from build123d import *

# Parameters (mm, degrees)
ESBO_O1_W                = 30
ESBO_O1_H                = 5
ESBO_O1_R                = 1.5
RESSALTO_EXTRUS_O1_DEPTH = 2
ESBO_O3_W                = 2
ESBO_O3_H                = 5
RESSALTO_EXTRUS_O2_DEPTH = 39
PADR_O_LINEAR1_COUNT     = 2
PADR_O_LINEAR1_PITCH     = 37
ESBO_O4_R                = 1.285304246
CORTE_EXTRUS_O1_DEPTH    = 39


with BuildPart() as part:
    # Esboço1 → Ressalto-extrusão1 (new body)
    with BuildSketch(Plane.XY):
        Rectangle(ESBO_O1_W, ESBO_O1_H)
        with Locations((-9, 0)):
            Circle(ESBO_O1_R, mode=Mode.SUBTRACT)
        with BuildLine():
            ThreePointArc((6, 1.118033989), (3.5, 0), (6, -1.118033989))
            ThreePointArc((6, -1.118033989), (7, -1.5), (8, -1.118033989))
            ThreePointArc((8, -1.118033989), (9, -1.5), (10, -1.118033989))
            ThreePointArc((10, -1.118033989), (12.5, 0), (10, 1.118033989))
            ThreePointArc((10, 1.118033989), (9, 1.5), (8, 1.118033989))
            ThreePointArc((8, 1.118033989), (7, 1.5), (6, 1.118033989))
        make_face(mode=Mode.SUBTRACT)
    ressalto_extrus_o1 = extrude(amount=RESSALTO_EXTRUS_O1_DEPTH)

    # Esboço3 → Ressalto-extrusão2 (add)
    with BuildSketch(Plane.XY.offset(2)):
        with Locations((16, 0)):
            Rectangle(ESBO_O3_W, ESBO_O3_H)
    ressalto_extrus_o2 = extrude(amount=-RESSALTO_EXTRUS_O2_DEPTH)

    # Padrão linear1: Ressalto-extrusão1 ×2
    with Locations(*[(0, 0, -i * PADR_O_LINEAR1_PITCH) for i in range(1, PADR_O_LINEAR1_COUNT)]):
        add(ressalto_extrus_o1)

    # Espelhar1: Ressalto-extrusão2 across plane
    add(ressalto_extrus_o2.mirror(Plane(origin=(0, 0, 0), x_dir=(0, 0, 1), z_dir=(1, 0, 0))))

    # Esboço4 → Corte-extrusão1 (cut)
    with BuildSketch(Plane(origin=(17, 0, 0), x_dir=(0, 0, -1), z_dir=(1, 0, 0))):
        with Locations((9, 0)):
            Circle(ESBO_O4_R)
        with Locations((26, 0)):
            Circle(ESBO_O4_R)
    extrude(amount=-CORTE_EXTRUS_O1_DEPTH, mode=Mode.SUBTRACT)


solid = part.part
Check sheet for the modelled part. Datum: model origin and axes. Units: mm. A direction names the side the tool comes from. Round coordinates to 2 decimals unless told otherwise and drop trailing zeros. Loops run counter-clockwise (first coordinate to the right, second up) from the corner with the lowest first, then second, coordinate; pieces in that order, holes last.
1. Sectioned sample at C-C on z = -4. Record the boundary of the cut face in (x, y).
2. Sectioned sample at A-A on x = -8. Record the boundary of the cut face in (y, z), and give its area (3 significant figures).
3. Set-up check for faces 4 (the flat face through (0, 0, -35)), 5 (the cylindrical face through (7, 1.5, -36)), 6 (the flat face through (15.2, 2.5, -16)): record each of +Z, -Z, +X, -X, +Y, -Y from which the full face is reachable in a straight line by a thin tool's end or side.
4. Mould release check, pull along Y, two halves, no side actions. Record for faces 1 (the cylindrical face through (9, -1.5, -36)), 2 (the flat face through (-17, 0, -17)), 3 (the flat face through (15.2, -2.5, -16)): released by +Y, released by -Y, zero draft, split by the parting line, or undercut.
5. Gauge pin test, flat ends, axial feed: pin 1 Ø2.5 at (x, y) = (5, 0) entering from +Z; pin 2 Ø10 at (x, z) = (10.5, -13) entering from +Y. Record the tip position at first contact, or that the pin passes through.
6. Scan lines: probe 1 along Z at (x, y) = (13, 0.6); probe 2 along Y at (x, z) = (5, 0.6); probe 3 along X at (y, z) = (-0.85, -27). Record each from-to range of solid material in increasing order.
7. Sectioned sample at D-D on y = 0. Give the number of separate pieces and of enclosed holes in the cut face, and give its area (3 significant figures).
8. Sectioned sample at B-B on z = -26. Record the boundary of the cut face in (x, y), and give its area (3 significant figures).
Recorded:
1. outline: (-17, -2.5) - (-15, -2.5) - (-15, 2.5) - (-17, 2.5) - close; (15, -2.5) - (17, -2.5) - (17, 2.5) - (15, 2.5) - close
2. outline: (-2.5, -37) - (-1.12, -37) - (-1.12, -35) - (-2.5, -35) - close; (-2.5, 0) - (-1.12, 0) - (-1.12, 2) - (-2.5, 2) - close; (1.12, -37) - (2.5, -37) - (2.5, -35) - (1.12, -35) - close; (1.12, 0) - (2.5, 0) - (2.5, 2) - (1.12, 2) - close
2. area: 11.1 mm2
3. face 4: +Y, -Y
3. face 5: +Z, -Z
3. face 6: +Z, -Z, +X, -X, +Y
4. face 1: undercut
4. face 2: zero draft
4. face 3: released by -Y
5. pin 1: passes through
5. pin 2: stops at y = 2.5
6. probe 1: z = -37 to -35, 0 to 2
6. probe 2: y = -2.5 to -1.5, 1.5 to 2.5
6. probe 3: x = -17 to -15, 15 to 17
7. separate pieces: 8
7. enclosed holes: 0
7. area: 207 mm2
8. outline: (-17, -2.5) - (-15, -2.5) - (-15, -1.29) - (-17, -1.29) - close; (-17, 1.29) - (-15, 1.29) - (-15, 2.5) - (-17, 2.5) - close; (15, -2.5) - (17, -2.5) - (17, -1.29) - (15, -1.29) - close; (15, 1.29) - (17, 1.29) - (17, 2.5) - (15, 2.5) - close
8. area: 9.72 mm2
